For this review, take the finished solid that the model builds, in its own axes (mm). Face numbers are marked on the shaded views. A direction names the side the tool comes from. Give positions to 0.01 mm unless a question says otherwise; leave off trailing zeros. Order: outer loops, then holes, each group sorted by start corner. A loop starts at its lowest first (then second) coordinate and runs counter-clockwise, first axis right, second up.
Item 1: For P1, Ø2, axis at x = 17.5, y = 20.5, coming from the -Z side; P2, Ø3, axis at x = 9, z = 29, coming from the +Y side; P3, Ø5, axis at x = -32.5, y = 14.5, coming from the -Z side (3 decimals); P4, Ø2, axis at x = 17, z = -25, coming from the -Y side, all flat-tipped, find the tip position at first contact; note any pin that passes through.
Item 2: Machinability: for the marked faces 1, 2 and 3, which of the approach directions +Z, -Z, +X, -X, +Y, -Y give a long, thin tool a straight path to every point of the face, cutting with its end or side? Answer none if there is none.
Item 3: Consider section A-A (z = -33). Give the boundary of the cut face in (x, y).
Item 4: Consider section B-B (y = 31). Give the boundary of the cut face in (x, z).
Item 5: For probe 1 along Y at (x, z) = (-16, 21); probe 2 along Y at (x, z) = (44.5, 19); probe 3 along Z at (x, y) = (33.5, 12), list the stretches that pass through material, from the lowest coordinate up.
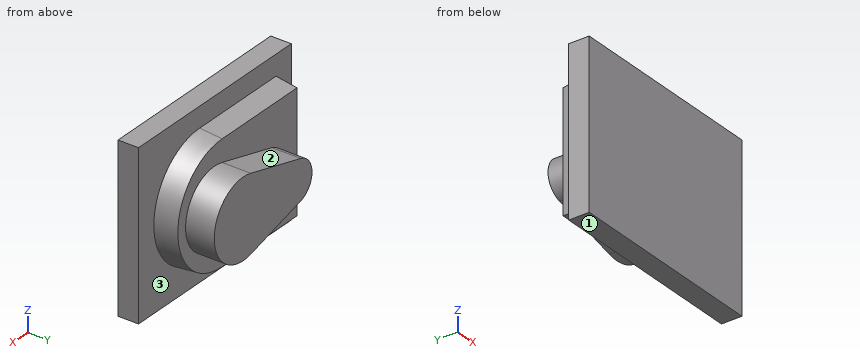
```python
from build123d import *

# Parameters (mm, degrees)
SKETCH_1_W      = 100
SKETCH_1_H      = 80
EXTRUDE_1_DEPTH = 10
EXTRUDE_2_DEPTH = 11
EXTRUDE_2_TAPER = 5
EXTRUDE_3_DEPTH = 14


with BuildPart() as part:
    # 스케치1 → 보스-돌출1 (new body)
    with BuildSketch(Plane(origin=(0, 0, 0), x_dir=(1, 0, 0), z_dir=(0, 1, 0))):
        Rectangle(SKETCH_1_W, SKETCH_1_H)
    extrude(amount=EXTRUDE_1_DEPTH)

    # 스케치2 → 보스-돌출2 (add)
    with BuildSketch(Plane(origin=(0, 10, 0), x_dir=(1, 0, 0), z_dir=(0, 1, 0))):
        with BuildLine():
            Line((10, 30), (-40, 30))
            Line((-40, 30), (-40, -30))
            Line((-40, -30), (10, -30))
            ThreePointArc((10, -30), (40, 0), (10, 30))
        make_face()
    extrude(amount=EXTRUDE_2_DEPTH, taper=EXTRUDE_2_TAPER)

    # 스케치3 → 보스-돌출3 (add)
    with BuildSketch(Plane(origin=(0, 21, 0), x_dir=(1, 0, 0), z_dir=(0, 1, 0))):
        with BuildLine():
            Line((-22.571428571, 9.663734014), (10.114285714, 18.361094627))
            ThreePointArc((10.114285714, 18.361094627), (34, 0), (10.114285714, -18.361094627))
            Line((10.114285714, -18.361094627), (-22.571428571, -9.663734014))
            ThreePointArc((-22.571428571, -9.663734014), (-30, 0), (-22.571428571, 9.663734014))
        make_face()
    extrude(amount=EXTRUDE_3_DEPTH)


solid = part.part
```
Resolved:
1. P1: stops at z = -28.36
1. P2: stops at y = 21
1. P3: stops at z = -29.825
1. P4: stops at y = 0
2. face 1: -Z, +X, -X, +Y, -Y
2. face 2: +Z, -X, +Y
2. face 3: +Y
3. outline: (-50, 0) - (50, 0) - (50, 10) - (-50, 10) - close
4. outline: (-22.57, -9.66) - (10.11, -18.36) arc R19 ccw (long way) to (10.11, 18.36) - (-22.57, 9.66) arc R10 ccw to start
5. probe 1: y = 0 to 21
5. probe 2: y = 0 to 10
5. probe 3: z = -18.37 to 18.37
